Here's the drawing with two shaded views (mm, measured from the low corner). I have some questions. A direction names the side the tool comes from. Give positions to 0.01 mm unless a question says otherwise; leave off trailing zeros. Loops run counter-clockwise (first coordinate to the right, second up) from the corner with the lowest first, then second, coordinate; pieces in that order, holes last. Notation, with made-up numbers: (-13, 38.25) -> (2, 38.25) arc R7 cw to (2, 42.25) -> close; hole circle Ø8 at (16.5, 47). An arc over 180 degrees is marked (long way). Put each result on its own line as item: value.
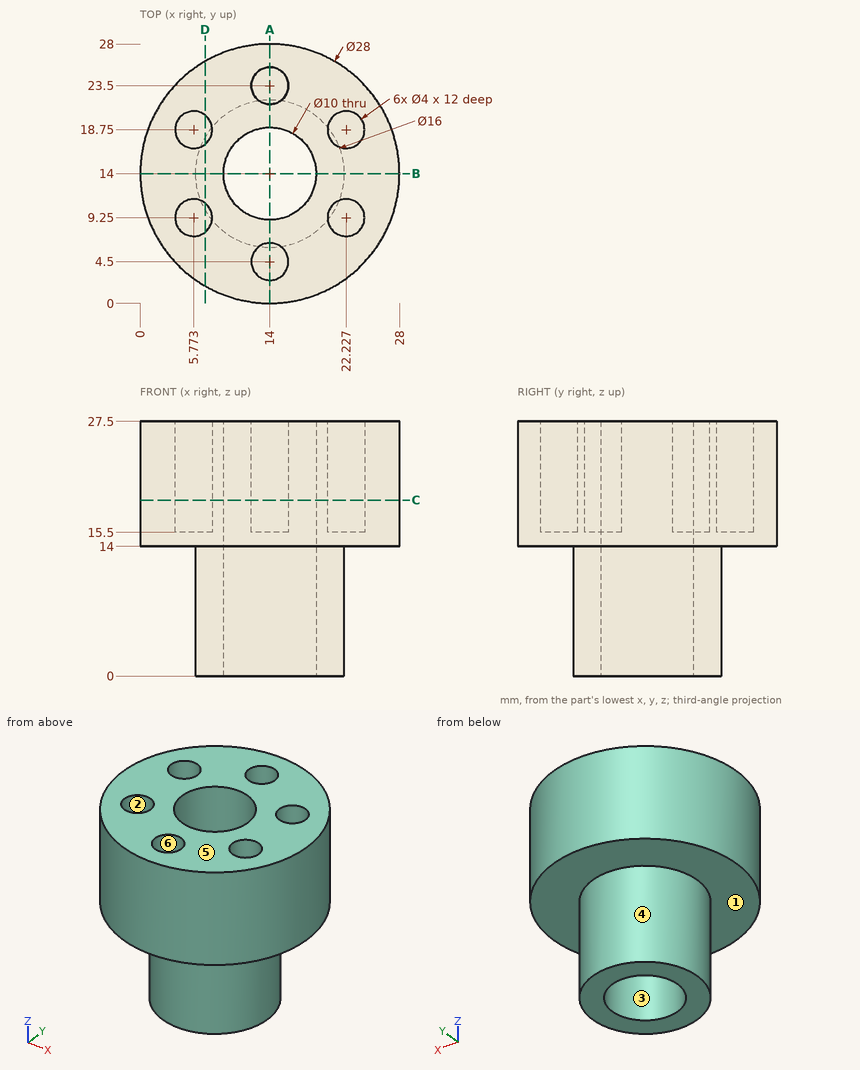
1. If we section it at D-D (x = 7): List the corners of the cut face in (y, z) for me.
Recorded:
outline: (1.88, 14) -> (10.13, 14) -> (10.13, 0) -> (17.87, 0) -> (17.87, 14) -> (26.12, 14) -> (26.12, 27.5) -> (20.33, 27.5) -> (20.33, 15.5) -> (17.17, 15.5) -> (17.17, 27.5) -> (10.83, 27.5) -> (10.83, 15.5) -> (7.67, 15.5) -> (7.67, 27.5) -> (1.88, 27.5) -> close
2. For the marked faces 1, 2 and 3, which set-ups out of +Z, -Z, +X, -X, +Y, -Y let a thin tool reach every point of the face, with its end or its side?
Recorded:
face 1: -Z
face 2: +Z
face 3: +Z, -Z
3. If we section it at A-A (x = 14): List the corners of the cut face in (y, z) for me.
Recorded:
outline: (0, 14) -> (6, 14) -> (6, 0) -> (9, 0) -> (9, 27.5) -> (6.5, 27.5) -> (6.5, 15.5) -> (2.5, 15.5) -> (2.5, 27.5) -> (0, 27.5) -> close; (19, 0) -> (22, 0) -> (22, 14) -> (28, 14) -> (28, 27.5) -> (25.5, 27.5) -> (25.5, 15.5) -> (21.5, 15.5) -> (21.5, 27.5) -> (19, 27.5) -> close
4. If we section it at B-B (y = 14): List the corners of the cut face in (x, z) for me, then the cut area to 3 significant figures.
Recorded:
outline: (0, 14) -> (6, 14) -> (6, 0) -> (9, 0) -> (9, 27.5) -> (0, 27.5) -> close; (19, 0) -> (22, 0) -> (22, 14) -> (28, 14) -> (28, 27.5) -> (19, 27.5) -> close
area: 327 mm^2
5. I need wall thicknesses on line 1 (Y direction, x = 14, z = 24.75); line 2 (Y direction, x = 20.75, z = 24.5) (1 decimal); line 3 (Z direction, x = 23.5, y = 21.25). Which ranges of each line are inside material? Lowest first, please.
Recorded:
line 1: y = 0 to 2.5, 6.5 to 9, 19 to 21.5, 25.5 to 28
line 2: y = 1.7 to 7.9, 10.6 to 17.4, 20.1 to 26.3
line 3: z = 14 to 27.5
6. If we section it at C-C (z = 19): List the corners of the cut face in (x, y) for me.
Recorded:
outline: circle Ø28 at (14, 14); hole circle Ø4 at (5.77, 9.25); hole circle Ø4 at (5.77, 18.75); hole circle Ø10 at (14, 14); hole circle Ø4 at (14, 4.5); hole circle Ø4 at (14, 23.5); hole circle Ø4 at (22.23, 9.25); hole circle Ø4 at (22.23, 18.75)
7. Thinking about a two-plate mould opening in X: for the marked faces 4, 5 and 6, which applies, pulls with the +X half, pulls with the -X half, needs draft (parallel to the pull), parting line crosses it, or undercut?
Recorded:
face 4: parting line crosses it
face 5: needs draft
face 6: undercut
8. I'm going to push flat-ended pins straight in: pin 1 (6 mm diameter, centred on x = 22.5, y = 6.5, fed in from -Z); pin 2 (4.5 mm diameter, centred on x = 5.77, y = 9.25, fed in from +Z); pin 3 (9 mm diameter, centred on x = 14, y = 14, fed in from -Z); pin 4 (3 mm diameter, centred on x = 5.77, y = 18.75, fed in from +Z). Where does each tip first touch, or does it pass through?
Recorded:
pin 1: stops at z = 14
pin 2: stops at z = 27.5
pin 3: passes through
pin 4: stops at z = 15.5
